Build history of the part. All positions in model axes, mm. Give positions to 0.01 mm unless a question says otherwise; leave off trailing zeros. Answer in a Markdown table with one row per item.
```python
from build123d import *

# Parameters (mm, degrees)
SKETCH1_R           = 49.53
SKETCH1_R_2         = 46.99
BOSS_EXTRUDE1_DEPTH = 182.88
CUT_EXTRUDE1_DEPTH  = 177.8
SKETCH3_R           = 49.53
SKETCH3_R_2         = 46.99
BOSS_EXTRUDE2_DEPTH = 2.54
SKETCH4_R           = 49.53
SKETCH4_R_2         = 46.99
BOSS_EXTRUDE3_DEPTH = 2.54
BOSS_EXTRUDE4_START = -5.08
SKETCH5_R           = 49.53
BOSS_EXTRUDE4_DEPTH = 5.08
SKETCH6_W           = 50.419
SKETCH6_H           = 4.699
BOSS_EXTRUDE5_DEPTH = 2.54
SKETCH7_R           = 0.8255
BOSS_EXTRUDE6_DEPTH = 2.54
CIRPATTERN2_COUNT   = 8


with BuildPart() as part:
    # Sketch1 → Boss-Extrude1 (new, symmetric)
    with BuildSketch(Plane(origin=(0, 0, 0), x_dir=(1, 0, 0), z_dir=(0, 1, 0))):
        with Locations(Location((0, 0, 0), (0, 0, 270))):
            Circle(SKETCH1_R)
        with Locations(Location((0, 0, 0), (0, 0, 270))):
            Circle(SKETCH1_R_2, mode=Mode.SUBTRACT)
    extrude(amount=BOSS_EXTRUDE1_DEPTH, both=True)

    # Sketch2 → Cut-Extrude1 (cut, symmetric)
    with BuildSketch(Plane(origin=(0, 0, 0), x_dir=(1, 0, 0), z_dir=(0, 1, 0))):
        with BuildLine():
            Line((34.339077963, -32.07628134), (36.13611782, -33.873321197))
            ThreePointArc((36.13611782, -33.873321197), (45.710930003, -19.071753413), (49.49527883, -1.854258207))
            Line((49.49527883, -1.854258207), (46.953400585, -1.854258207))
            ThreePointArc((46.953400585, -1.854258207), (43.364264524, -18.099742051), (34.339077963, -32.07628134))
        make_face()
        with BuildLine():
            ThreePointArc((1.584890151, -49.504636381), (18.664975227, -45.878530924), (33.425440685, -36.550797734))
            Line((33.425440685, -36.550797734), (31.627502039, -34.752859088))
            ThreePointArc((31.627502039, -34.752859088), (17.692915235, -43.531837205), (1.584890151, -46.963264614))
            Line((1.584890151, -46.963264614), (1.584890151, -49.504636381))
        make_face()
        with BuildLine():
            ThreePointArc((-33.543952964, -36.442065248), (-19.03558139, -45.726005086), (-2.225109849, -49.479993797))
            Line((-2.225109849, -49.479993797), (-2.225109849, -46.937287801))
            ThreePointArc((-2.225109849, -46.937287801), (-18.063572268, -43.379343666), (-31.746279167, -34.644391451))
            Line((-31.746279167, -34.644391451), (-33.543952964, -36.442065248))
        make_face()
        with BuildLine():
            Line((46.949282998, 1.955741793), (49.491372723, 1.955741793))
            ThreePointArc((49.491372723, 1.955741793), (45.777644234, 18.911059948), (36.442065248, 33.543952964))
            Line((36.442065248, 33.543952964), (34.644391451, 31.746279167))
            ThreePointArc((34.644391451, 31.746279167), (43.430990742, 17.93903964), (46.949282998, 1.955741793))
        make_face()
        with BuildLine():
            ThreePointArc((-49.49527883, -1.854258207), (-45.741824116, -18.997537381), (-36.245883162, -33.755841773))
            Line((-36.245883162, -33.755841773), (-34.448634556, -31.958593167))
            ThreePointArc((-34.448634556, -31.958593167), (-43.39516767, -18.025524205), (-46.953400585, -1.854258207))
            Line((-46.953400585, -1.854258207), (-49.49527883, -1.854258207))
        make_face()
        with BuildLine():
            Line((31.958593167, 34.448634556), (33.755841773, 36.245883162))
            ThreePointArc((33.755841773, 36.245883162), (18.873008967, 45.79334485), (1.584890151, 49.504636381))
            Line((1.584890151, 49.504636381), (1.584890151, 46.963264614))
            ThreePointArc((1.584890151, 46.963264614), (17.900986276, 43.446689061), (31.958593167, 34.448634556))
        make_face()
        with BuildLine():
            ThreePointArc((-36.550797734, 33.425440685), (-45.80828813, 18.836709868), (-49.491372723, 1.955741793))
            Line((-49.491372723, 1.955741793), (-46.949282998, 1.955741793))
            ThreePointArc((-46.949282998, 1.955741793), (-43.461630715, 17.864678995), (-34.752859088, 31.627502039))
            Line((-34.752859088, 31.627502039), (-36.550797734, 33.425440685))
        make_face()
        with BuildLine():
            Line((-2.225109849, 46.937287801), (-2.225109849, 49.479993797))
            ThreePointArc((-2.225109849, 49.479993797), (-19.242893169, 45.63914945), (-33.873321197, 36.13611782))
            Line((-33.873321197, 36.13611782), (-32.07628134, 34.339077963))
            ThreePointArc((-32.07628134, 34.339077963), (-18.270880717, 43.292436035), (-2.225109849, 46.937287801))
        make_face()
    extrude(amount=CUT_EXTRUDE1_DEPTH, both=True, mode=Mode.SUBTRACT)

    # Sketch3 → Boss-Extrude2 (add, symmetric)
    with BuildSketch(Plane(origin=(0, 91.44, 0), x_dir=(1, 0, 0), z_dir=(0, 1, 0))):
        with Locations(Location((0, 0, 0), (0, 0, 270))):
            Circle(SKETCH3_R)
        with Locations(Location((0, 0, 0), (0, 0, 270))):
            Circle(SKETCH3_R_2, mode=Mode.SUBTRACT)
    boss_extrude2 = extrude(amount=BOSS_EXTRUDE2_DEPTH, both=True)

    # Mirror1: Boss-Extrude2 across plane
    add(boss_extrude2.mirror(Plane.ZX))

    # Sketch4 → Boss-Extrude3 (add, symmetric)
    with BuildSketch(Plane(origin=(0, 0, 0), x_dir=(1, 0, 0), z_dir=(0, 1, 0))):
        with Locations(Location((0, 0, 0), (0, 0, 270))):
            Circle(SKETCH4_R)
        with Locations(Location((0, 0, 0), (0, 0, 270))):
            Circle(SKETCH4_R_2, mode=Mode.SUBTRACT)
    extrude(amount=BOSS_EXTRUDE3_DEPTH, both=True)

    # Sketch5 → Boss-Extrude4 (add)
    with BuildSketch(Plane.XZ.offset(182.88).offset(BOSS_EXTRUDE4_START)):
        with Locations(Location((0, 0, 0), (0, 0, 90))):
            Circle(SKETCH5_R)
    extrude(amount=BOSS_EXTRUDE4_DEPTH)

    # Sketch6 → Boss-Extrude5 (add)
    with BuildSketch(Plane(origin=(0, -177.8, 0), x_dir=(1, 0, 0), z_dir=(0, 1, 0))):
        Rectangle(SKETCH6_W, SKETCH6_H)
    extrude(amount=BOSS_EXTRUDE5_DEPTH)

    # Sketch7 → Boss-Extrude6 (add)
    with BuildSketch(Plane(origin=(0, 182.88, 0), x_dir=(1, 0, 0), z_dir=(0, 1, 0))):
        with Locations(Location((48.26, 0, 0), (0, 0, 270))):
            Circle(SKETCH7_R)
    boss_extrude6 = extrude(amount=BOSS_EXTRUDE6_DEPTH)

    # CirPattern2: Boss-Extrude6 ×8 about axis
    cirpattern2_axis = Axis((0, 0, 0), (0, 1, 0))
    for i in range(1, CIRPATTERN2_COUNT):
        add(boss_extrude6.rotate(cirpattern2_axis, i * 360 / CIRPATTERN2_COUNT))


solid = part.part
```
1. Drop flat-ended pins along their axis: P1, Ø7.5, axis at x = -17, z = -38.5, coming from the +Y side; P2, Ø6, axis at y = 80.5, z = 3, coming from the +X side; P3, Ø4.5, axis at x = 44, z = 17, coming from the +Y side. Give the stop position or say it passes through.
Check result:
| item | result |
|---|---|
| P1 | stops at y = -177.8 |
| P2 | stops at x = 49.53 |
| P3 | stops at y = 182.88 |
2. Probe line 1 (X direction, y = 22, z = 0); line 2 (Y direction, x = 14, z = -14). List the from-to ranges inside material, lowest first.
Check result:
| item | result |
|---|---|
| line 1 | x = -49.53 to -46.99, 46.99 to 49.53 |
| line 2 | y = -182.88 to -177.8 |
3. Cut at A-A on y = -71. Count the separate pieces of the cut face and the enclosed holes in it, and give its area (3 significant figures).
Check result:
| item | result |
|---|---|
| separate pieces | 8 |
| enclosed holes | 0 |
| area | 77.4 mm² |
4. Two-plate mould, pull along X, no slides. Class faces 1 (the face through (44, -88.9, 18)), 2 (the face through (-1, -177.8, 10)): +X half, -X half, draft (parallel to the pull), parting line (faces both ways), or undercut.
Check result:
| item | result |
|---|---|
| face 1 | draft |
| face 2 | undercut |
